from build123d import *

# Parameters (mm, degrees)
SKETCH_1_W      = 4
SKETCH_1_H      = 4
EXTRUDE_1_DEPTH = 36
SKETCH_3_R      = 1
EXTRUDE_2_DEPTH = 8


with BuildPart() as part:
    # 草图1 → 凸台-拉伸1 (new body)
    with BuildSketch(Plane.XY):
        Rectangle(SKETCH_1_W, SKETCH_1_H)
    extrude(amount=EXTRUDE_1_DEPTH)

    # 草图3 → 凸台-拉伸2 (add, symmetric)
    with BuildSketch(Plane(origin=(0, 0, 0), x_dir=(1, 0, 0), z_dir=(0, 1, 0))):
        with Locations((1, 0)):
            Circle(SKETCH_3_R)
    extrude(amount=EXTRUDE_2_DEPTH, both=True)


solid = part.part
Could you check a few things on this model? Use its own coordinates, in mm. A direction names the side the tool comes from. Round coordinates to 2 decimals unless told otherwise and drop trailing zeros. Order: outer loops, then holes, each group sorted by start corner. A loop starts at its lowest first (then second) coordinate and runs counter-clockwise, first axis right, second up.
(1) Please list where these lines run through material, in increasing order: line 1 along Y through (x, z) = (1.25, 9.5); line 2 along Z through (x, y) = (1.1, 5.5); line 3 along Z through (x, y) = (-1.5, 1.25).
Response values:
line 1: y = -2 to 2
line 2: z = -0.99 to 0.99
line 3: z = 0 to 36
(2) Imagine slicing it at C-C (z = 25). Write out the boundary of the cut face in (x, y).
Response values:
outline: (-2, -2) - (2, -2) - (2, 2) - (-2, 2) - close
(3) Imagine slicing it at B-B (y = 1). Write out the boundary of the cut face in (x, z).
Response values:
outline: (-2, 0) - (0, 0) arc R1 ccw to (2, 0) - (2, 36) - (-2, 36) - close
(4) Imagine slicing it at D-D (x = -1.45). Write out the boundary of the cut face in (y, z), plus the area to 3 significant figures.
Response values:
outline: (-2, 0) - (2, 0) - (2, 36) - (-2, 36) - close
area: 144 mm2
(5) Which directions (+Z, -Z, +X, -X, +Y, -Y) give clear straight access to the entire face, cutting with the end or side of a thin tool? Please do faces 1 (the flat face through (-1, 0, 0)), 2 (the flat face through (1, -8, 0)), 3 (the cylindrical face through (1, 0, -1)).
Response values:
face 1: -Z, -X, +Y, -Y
face 2: +Z, -Z, +X, -X, -Y
face 3: none
(6) Imagine slicing it at A-A (x = 1.6). Write out the boundary of the cut face in (y, z).
Response values:
outline: (-8, -0.8) - (8, -0.8) - (8, 0.8) - (2, 0.8) - (2, 36) - (-2, 36) - (-2, 0.8) - (-8, 0.8) - close
(7) I'm going to push flat-ended pins straight in: pin 1 (1 mm diameter, centred on x = -0.5, z = 17, fed in from +Y); pin 2 (6 mm diameter, centred on y = 6, z = 29, fed in from -X); pin 3 (1 mm diameter, centred on x = -1.5, y = 0, fed in from -Z); pin 4 (2 mm diameter, centred on x = 1, y = 3.5, fed in from +Z). Where does each tip first touch, or does it pass through?
Response values:
pin 1: stops at y = 2
pin 2: passes through
pin 3: stops at z = 0
pin 4: stops at z = 1
